Work out the finished part from the listing and answer in its coordinate system (mm). Give positions to 0.01 mm unless a question says otherwise; leave off trailing zeros. Loops run counter-clockwise (first coordinate to the right, second up) from the corner with the lowest first, then second, coordinate; pieces in that order, holes last. Notation, with made-up numbers: M 50.25,59.25 L 98.25,59.25 A30 cw 98.25,94.25 Z; hole C 37,-15.75 d7. An arc over 180 degrees is marked long. Answer as a JSON object with one key per item and string values. Group by question number.
```python
from build123d import *

# Parameters (mm, degrees)
SKETCH1_W                = 0.5
SKETCH1_H                = 20
BOSS_EXTRUDE1_DEPTH      = 2.4
BOSS_EXTRUDE2_DEPTH      = 0.5
BOSS_EXTRUDE2_DEPTH_BACK = 2.9
SKETCH2_R                = 0.2
CUT_EXTRUDE1_REACH       = 22.215


with BuildPart() as part:
    # Sketch1 → Boss-Extrude1 (new body)
    with BuildSketch(Plane.XY):
        with Locations((0, 10)):
            Rectangle(SKETCH1_W, SKETCH1_H)
    extrude(amount=BOSS_EXTRUDE1_DEPTH)

    # Sketch2 → Boss-Extrude2 (add, two sides: drawn at the far end of the back side and taken through both)
    with BuildSketch(Plane.XY.offset(2.4).offset(-BOSS_EXTRUDE2_DEPTH_BACK)):
        Circle(SKETCH2_R)
    extrude(amount=BOSS_EXTRUDE2_DEPTH + BOSS_EXTRUDE2_DEPTH_BACK)

    # Sketch3 → Cut-Extrude1 (cut, up to next)
    with BuildSketch(Plane(origin=(0.25, 0, 0), x_dir=(0, 0, -1), z_dir=(1, 0, 0)), mode=Mode.PRIVATE) as cut_extrude1_sk1:
        Polygon((-2.4, 0.3), (-3.130095712, 0.3), (-3.130095712, 41.705801687), (-0.2, 41.705801687), (-0.2, 20), (-2.188257625, 17.630486832), align=None)
    cut_extrude1_tool1 = extrude(cut_extrude1_sk1.sketch, amount=-CUT_EXTRUDE1_REACH, mode=Mode.PRIVATE) & part.part
    add(cut_extrude1_tool1.solids().sort_by_distance((0.25, 26.424814, 1.871))[0], mode=Mode.SUBTRACT)


solid = part.part
```
Item 1: A cutting plane is placed at B-B (y = 12.75). Determine the outline of the cut face in (x, z), and give its area (3 significant figures).
Item 2: A cutting plane is placed at C-C (y = 3). Determine the outline of the cut face in (x, z).
Item 3: Find the intervals of material crossed by probe 1 along Z at (x, y) = (0.05, 17.5); probe 2 along Y at (x, z) = (0, -0.3); probe 3 along Y at (x, z) = (-0.15, 1.7), in increasing order. Write a range as [from, to].
Item 4: A cutting plane is placed at A-A (x = 0). Determine the outline of the cut face in (y, z), and give its area (3 significant figures).
The answers:
{
 "1": {"outline": "M -0.25,0 L 0.25,0 L 0.25,2.25 L -0.25,2.25 Z", "area": "1.12 mm^2"},
 "2": {"outline": "M -0.25,0 L 0.25,0 L 0.25,2.37 L -0.25,2.37 Z"},
 "3": {"probe 1": "z = [0, 2.19]", "probe 2": "y = [-0.2, 0.2]", "probe 3": "y = [-0.13, 18.21]"},
 "4": {"outline": "M -0.2,-0.5 L 0.2,-0.5 L 0.2,0 L 20,0 L 20,0.2 L 17.63,2.19 L 0.3,2.4 L 0.2,2.4 L 0.2,2.9 L -0.2,2.9 Z", "area": "44.2 mm^2"}
}
